Model file for the job. Use its own axes, mm. A direction names the side the tool comes from. Give positions to 0.01 mm unless a question says otherwise; leave off trailing zeros. Order: outer loops, then holes, each group sorted by start corner. A loop starts at its lowest first (then second) coordinate and runs counter-clockwise, first axis right, second up. Notation, with made-up numbers: M 23,-35 L 47,-35 A30 ccw 47,-2 Z; hole C 59.25,61 d10. An arc over 180 degrees is marked long. Return JSON: item names as keys, results as strings. Group by question number.
1. Slice it at B-B on x = 0. List the corners of the cut face in (y, z).
2. Slice it at C-C on z = 0. List the corners of the cut face in (x, y).
3. Slice it at D-D on x = 3.75. List the corners of the cut face in (y, z), then the cut area to 3 significant figures.
4. Wall check: probe 1 along Z at (x, y) = (-3.75, 43.5); probe 2 along Z at (x, y) = (-1, 4.5); probe 3 along X at (y, z) = (31.5, 4). Give the ranges that are in metal, low to high. Write a range as [from, to].
5. 3-axis set-ups, long thin cutter, end or side, ignore diameter. For faces 5 (the face through (-1.5, 3, 0)), 6 (the face through (0, 46, 2.5)), 7 (the face through (-2, 0, 0)), 8 (the face through (0, 46, -2.5)): which of +Z, -Z, +X, -X, +Y, -Y reach the whole face in a straight line?
6. Pin check, flat tips, straight feed: pin 1 (1.5 mm diameter, centred on y = 7, z = -2, fed in from +X); pin 2 (2 mm diameter, centred on y = 28, z = -1, fed in from +X); pin 3 (2.5 mm diameter, centred on x = -2, y = 47, fed in from +Z); pin 4 (6 mm diameter, centred on x = 3.5, z = 0.5, fed in from +Y). Stop position of each tip, or through.
7. Two-plate mould, pull along X, no slides. Class faces 1 (the face through (-0.061, 41.249, 2.904)), 2 (the face through (0, 55, 0)), 3 (the face through (0, 6, 0)), 4 (the face through (0, 53, 0)): released by +X, released by -X, zero draft, split by the parting line, or undercut.
8. Slice it at A-A on y = 50. List the corners of the cut face in (x, z), then the cut area to 3 significant figures.
from build123d import *

# Parameters (mm, degrees)
SKETCH1_R               = 5
BOSS_EXTRUDE1_DEPTH     = 55
CUT_EXTRUDE2_DEPTH      = 56.452682532
CUT_EXTRUDE2_DEPTH_BACK = 56.452682532
SKETCH6_R               = 3
CUT_EXTRUDE3_DEPTH      = 56.733742145
CUT_EXTRUDE4_DEPTH      = 56.733742145
CUT_EXTRUDE5_DEPTH      = 6


with BuildPart() as part:
    # Sketch1 → Boss-Extrude1 (new body)
    with BuildSketch(Plane(origin=(0, 0, 0), x_dir=(1, 0, 0), z_dir=(0, 1, 0))):
        with Locations(Location((0, 0, 0), (0, 0, 270))):
            Circle(SKETCH1_R)
    extrude(amount=BOSS_EXTRUDE1_DEPTH)

    # Sketch5 → Cut-Extrude2 (cut, two sides: drawn at the far end of the back side and taken through both)
    with BuildSketch(Plane(origin=(0, 0, 0), x_dir=(0, 0, -1), z_dir=(1, 0, 0)).offset(-CUT_EXTRUDE2_DEPTH_BACK)):
        with BuildLine():
            Line((-2.5, 55), (-2.5, 43))
            ThreePointArc((-2.5, 43), (-3.671572875, 40.171572875), (-6.5, 39))
            Line((-6.5, 39), (-6.5, 55))
            Line((-6.5, 55), (-2.5, 55))
        make_face()
        with BuildLine():
            Line((6.5, 55), (6.5, 39))
            ThreePointArc((6.5, 39), (3.671572875, 40.171572875), (2.5, 43))
            Line((2.5, 43), (2.5, 55))
            Line((2.5, 55), (6.5, 55))
        make_face()
    extrude(amount=CUT_EXTRUDE2_DEPTH + CUT_EXTRUDE2_DEPTH_BACK, mode=Mode.SUBTRACT)

    # Sketch6 → Cut-Extrude3 (cut, through all)
    with BuildSketch(Plane.XY.offset(2.5)):
        with Locations((0, 50)):
            Circle(SKETCH6_R)
    extrude(amount=-CUT_EXTRUDE3_DEPTH, mode=Mode.SUBTRACT)

    # Sketch7 → Cut-Extrude4 (cut, through all)
    with BuildSketch(Plane(origin=(0, 0, -2.5), x_dir=(-1, 0, 0), z_dir=(0, 0, -1))):
        with BuildLine():
            Line((-4.829629131, 51.294095226), (-10.892994719, 28.665306789))
            Line((-10.892994719, 28.665306789), (-10.892994719, 70.083373649))
            Line((-10.892994719, 70.083373649), (10.892994719, 70.083373649))
            Line((10.892994719, 70.083373649), (10.892994719, 28.665306789))
            Line((10.892994719, 28.665306789), (4.829629131, 51.294095226))
            ThreePointArc((4.829629131, 51.294095226), (0, 55), (-4.829629131, 51.294095226))
        make_face()
    extrude(amount=-CUT_EXTRUDE4_DEPTH, mode=Mode.SUBTRACT)

    # Sketch8 → Cut-Extrude5 (cut)
    with BuildSketch(Plane.XZ):
        with BuildLine():
            Line((-1.5, 2), (-1.5, -2))
            ThreePointArc((-1.5, -2), (0, -2.5), (1.5, -2))
            Line((1.5, -2), (1.5, 2))
            ThreePointArc((1.5, 2), (0, 2.5), (-1.5, 2))
        make_face()
    extrude(amount=-CUT_EXTRUDE5_DEPTH, mode=Mode.SUBTRACT)


solid = part.part
Result:
{
 "1": {"outline": "M 0,-5 L 39.29,-5 A4 cw 43,-2.5 L 47,-2.5 L 47,2.5 L 43,2.5 A4 cw 39.29,5 L 0,5 L 0,2.5 L 6,2.5 L 6,-2.5 L 0,-2.5 Z; M 53,-2.5 L 55,-2.5 L 55,2.5 L 53,2.5 Z"},
 "2": {"outline": "M -5,0 L -1.5,0 L -1.5,6 L 1.5,6 L 1.5,0 L 5,0 L 5,50.66 L 4.83,51.29 A5 ccw -4.83,51.29 L -5,50.66 Z; hole C 0,50 d6"},
 "3": {"outline": "M 0,-3.31 L 40.59,-3.31 A4 cw 43,-2.5 L 53.31,-2.5 L 53.31,2.5 L 43,2.5 A4 cw 40.59,3.31 L 0,3.31 Z", "area": "333 mm2"},
 "4": {"probe 1": "z = [-2.5, 2.5]", "probe 2": "z = [-4.9, -2.29], [2.29, 4.9]", "probe 3": "x = [-3, 3]"},
 "5": {"face 5": "-Y", "face 6": "+Z, +X, -X, +Y", "face 7": "+Z, -Z, +X, -X, -Y", "face 8": "-Z, +X, -X, +Y"},
 "6": {"pin 1": "stops at x = 4.84", "pin 2": "stops at x = 5", "pin 3": "stops at z = 2.5", "pin 4": "stops at y = 54.97"},
 "7": {"face 1": "zero draft", "face 2": "split by the parting line", "face 3": "undercut", "face 4": "undercut"},
 "8": {"outline": "M -4.33,-2.5 L -3,-2.5 L -3,2.5 L -4.33,2.5 A5 ccw Z; M 3,-2.5 L 4.33,-2.5 A5 ccw 4.33,2.5 L 3,2.5 Z", "area": "17.8 mm2"}
}
